Verification items for the finished model (mm, model axes). A direction names the side the tool comes from. Coordinates: 2 decimals unless noted, no trailing zeros. Order: outer loops, then holes, each group sorted by start corner. A loop starts at its lowest first (then second) coordinate and runs counter-clockwise, first axis right, second up. Notation, with made-up numbers: M 73,42 L 93,42 A28 cw 93,64 Z; hole C 25.5,55.25 d5. An arc over 180 degrees is marked long. Return JSON: item names as keys, results as strings. Group by question number.
Q1. Section check A-A, the plane y = 4.8. Enter the section's corners in (x, z) (3 decimals), then the cut area to 3 significant figures.
Q2. Access from +Z, -Z, +X, -X, +Y, -Y to the whole of each face (thin tool, end or side, straight path). Record for faces 4 (the face through (0.933, 1.578, 3.373)), 5 (the face through (-4.1, 5, 0)), 6 (the face through (6.5, 3, 0)).
Q3. Section check B-B, the plane z = 1.25. Enter the section's corners in (x, y) (3 decimals).
Q4. Section check C-C, the plane x = 1.25. Enter the section's corners in (y, z) (3 decimals), then the cut area to 3 significant figures.
Q5. Section check D-D, the plane y = 2.95. Enter the section's corners in (x, z).
Q6. Thickness scan on probe 1 along Z at (x, y) = (0, 5.45) (3 decimals); probe 2 along Z at (x, y) = (-3.5, 4.7) (3 decimals). Record the ranges inside material, lowest first.
Q7. Mould release check, pull along X, two halves, no side actions. Record for faces 1 (the face through (-3.388, 1.578, -0.879)), 2 (the face through (-6.5, 3, 0)), 3 (the face through (6, 6, 0)): pulls with the +X half, pulls with the -X half, needs draft (parallel to the pull), parting line crosses it, or undercut.
Autodesk Inventor part; units mm, degrees
ref_plane "YZ Plane" through (0, 0, 0) normal (1, 0, 0) x (0, 1, 0)
ref_plane "XY Plane" through (0, 0, 0) normal (0, 0, 1) x (1, 0, 0)
ref_plane "作業平面2" through (0, 6, 0) normal (0, 1, 0) x (-1, 0, 0)
sketch "スケッチ3" plane through (0, 6, 0) normal (0, 1, 0) x (-1, 0, 0)
  line L0 (4.1, -4.1) -> (-4.1, -4.1)
  line L1 (-4.1, -4.1) -> (-4.1, 4.1)
  line L2 (-4.1, 4.1) -> (4.1, 4.1)
  line L3 (4.1, 4.1) -> (4.1, -4.1)
  line L4 (4.1, -4.1) -> (-4.1, 4.1) construction
  line L5 (-4.1, -4.1) -> (4.1, 4.1) construction
  line L6 (4.925, -4.925) -> (-4.925, -4.925)
  line L7 (-4.925, -4.925) -> (-4.925, 4.925)
  line L8 (-4.925, 4.925) -> (4.925, 4.925)
  line L9 (4.925, 4.925) -> (4.925, -4.925)
  line L10 (4.925, -4.925) -> (-4.925, 4.925) construction
  line L11 (-4.925, -4.925) -> (4.925, 4.925) construction
  point P0 (0, 0)
  point P1 (0, 0)
  dimension "d19" = 8.2
  dimension "d20" = 8.2
  dimension "d21" = 9.85
  dimension "d22" = 9.85
sketch "スケッチ1" plane through (0, 0, 0) normal (0, 1, 0) x (-1, 0, 0)
  line L0 (6.5, -6.5) -> (-6.5, 6.5) construction
  line L1 (-6.5, -6.5) -> (6.5, 6.5) construction
  line L2 (1.046, 3.9037) -> (3.9037, 1.046)
  line L3 (3.9037, 1.046) -> (2.8577, -2.8577)
  line L4 (2.8577, -2.8577) -> (-1.046, -3.9037)
  line L5 (-1.046, -3.9037) -> (-3.9037, -1.046)
  line L6 (-3.9037, -1.046) -> (-2.8577, 2.8577)
  line L7 (-2.8577, 2.8577) -> (1.046, 3.9037)
  line L8 (-6.5, -6.5) -> (6.5, -6.5)
  line L9 (6.5, -6.5) -> (6.5, 6.5)
  line L10 (6.5, 6.5) -> (-6.5, 6.5)
  line L11 (-6.5, 6.5) -> (-6.5, -6.5)
  line L12 (-6.5, -6.5) -> (6.5, 6.5) construction
  line L13 (6.5, -6.5) -> (-6.5, 6.5) construction
  circle A0 centre (0, 0) radius 2.125
  dimension "d33" = 7
  dimension "d34" = 13
  dimension "d35" = 13
  dimension "d36" = 4.25
extrude "押し出し8" add sketch "スケッチ1" along normal blind 6 contours L2 L3 L4 L5 L6 L7 | L11 L10 L9 L8 | A0
extrude "押し出し9" cut sketch "スケッチ3" against normal blind 2
extrude "押し出し10" cut sketch "スケッチ1" along normal blind 3.2 contours L2 L3 L4 L5 L6 L7
extrude "押し出し11" cut sketch "スケッチ1" along normal blind 6 contours A0
properties part number "pin_joint_plastic_ver2"
Numbers:
{
 "1": {"outline": "M -6.5,-6.5 L 6.5,-6.5 L 6.5,6.5 L -6.5,6.5 Z; M -4.1,-4.1 L 4.1,-4.1 L 4.1,4.1 L -4.1,4.1 Z; hole M -4.925,-4.925 L 4.925,-4.925 L 4.925,4.925 L -4.925,4.925 Z; hole C 0,0 d4.25", "area": "125 mm2"},
 "2": {"face 4": "-Y", "face 5": "+Y", "face 6": "+Z, -Z, +X, +Y, -Y"},
 "3": {"outline": "M -6.5,0 L -3.7,0 L -3.7,3.2 L -1.718,3.2 L -1.718,6 L -4.1,6 L -4.1,4 L -4.925,4 L -4.925,6 L -6.5,6 Z; M 1.718,3.2 L 3.288,3.2 L 3.288,0 L 6.5,0 L 6.5,6 L 4.925,6 L 4.925,4 L 4.1,4 L 4.1,6 L 1.718,6 Z"},
 "4": {"outline": "M 0,-6.5 L 6,-6.5 L 6,-4.925 L 4,-4.925 L 4,-4.1 L 6,-4.1 L 6,-1.718 L 3.2,-1.718 L 3.2,-3.7 L 0,-3.7 Z; M 0,3.288 L 3.2,3.288 L 3.2,1.718 L 6,1.718 L 6,4.1 L 4,4.1 L 4,4.925 L 6,4.925 L 6,6.5 L 0,6.5 Z", "area": "42.7 mm2"},
 "5": {"outline": "M -6.5,-6.5 L 6.5,-6.5 L 6.5,6.5 L -6.5,6.5 Z; hole M -3.9,1.05 L -2.86,-2.86 L 1.05,-3.9 L 3.9,-1.05 L 2.86,2.86 L -1.05,3.9 Z"},
 "6": {"probe 1": "z = -6.5 to -4.925, -4.1 to -2.125, 2.125 to 4.1, 4.925 to 6.5", "probe 2": "z = -6.5 to -4.925, -4.1 to 4.1, 4.925 to 6.5"},
 "7": {"face 1": "undercut", "face 2": "pulls with the -X half", "face 3": "needs draft"}
}
